The listing builds one solid part. Answer for the finished solid, in the listing's coordinates (mm). Give positions to 0.01 mm unless a question says otherwise; leave off trailing zeros. Loops run counter-clockwise (first coordinate to the right, second up) from the corner with the lowest first, then second, coordinate; pieces in that order, holes last. Notation, with made-up numbers: M 45,-31 L 60,-31 A21 ccw 60,-18 Z; hole C 56.5,1.25 d9. An arc over 180 degrees is marked long. One line per item, written item: value. Start each with the question number.
Q1. A cutting plane is placed at A-A, the plane x = -6. Determine the outline of the cut face in (y, z), and give its area (3 significant figures).
Q2. A cutting plane is placed at B-B, the plane y = -230. Determine the outline of the cut face in (x, z).
Q3. A cutting plane is placed at C-C, the plane z = 9. Determine the outline of the cut face in (x, y), and give its area (3 significant figures).
Q4. Consider L1, parallel to X at y = 451, z = 4; L2, parallel to Z at x = -18.5, y = 475.5. Determine where each line is inside the solid, lowest interval first.
from build123d import *

# Parameters (mm, degrees)
F0_W     = 50.8
F0_H     = 50.8
F0_W_2   = 41.275
F0_H_2   = 41.275
F1_DEPTH = 584.2
F3_DEPTH = 50.8
F4_R     = 5.08


with BuildPart() as f1:
    # F0 (on Front) → F1 (new body, symmetric)
    with BuildSketch(Plane.XZ):
        Rectangle(F0_W, F0_H)
        Rectangle(F0_W_2, F0_H_2, mode=Mode.SUBTRACT)
    extrude(amount=F1_DEPTH, both=True)

    # F2 (on face) → F3 (cut)
    with BuildSketch(Plane.YZ.offset(25.4)):
        Polygon((-584.2, 25.4), (-584.2, -25.4), (-535.14301, 25.4), align=None)
    extrude(amount=-F3_DEPTH, mode=Mode.SUBTRACT)

    # F4
    f4_edges = [f1.edges().sort_by_distance(p)[0] for p in [
        (-25.4, 24.528495, 25.4),
        (25.4, 24.528495, 25.4),
        (20.6375, 2.299546, -20.6375),
        (-20.6375, 2.299546, -20.6375),
        (-25.4, 0, -25.4),
        (25.4, 0, -25.4),
    ]]
    fillet(f4_edges, radius=F4_R)


solid = f1.part
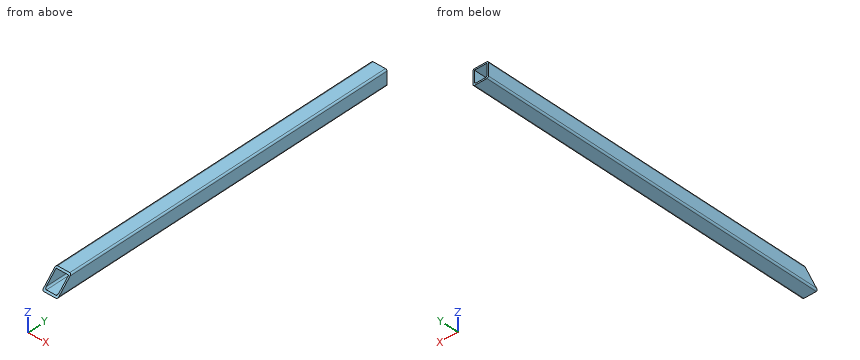
Answer block:
1. outline: M -584.2,-25.4 L 584.2,-25.4 L 584.2,-20.64 L -579.6,-20.64 Z; M -539.74,20.64 L 584.2,20.64 L 584.2,25.4 L -535.14,25.4 Z
1. area: 10,900 mm^2
2. outline: M -25.4,-20.32 A5.08 ccw -20.32,-25.4 L 20.32,-25.4 A5.08 ccw 25.4,-20.32 L 25.4,20.32 A5.08 ccw 20.32,25.4 L -20.32,25.4 A5.08 ccw -25.4,20.32 Z; hole M -20.64,-15.56 A5.08 ccw -15.56,-20.64 L 15.56,-20.64 A5.08 ccw 20.64,-15.56 L 20.64,20.64 L -20.64,20.64 Z
3. outline: M -25.4,-550.98 L -20.64,-550.98 L -20.64,584.2 L -25.4,584.2 Z; M 20.64,-550.98 L 25.4,-550.98 L 25.4,584.2 L 20.64,584.2 Z
3. area: 10,800 mm^2
4. L1: -25.4 to -20.64, 20.64 to 25.4
4. L2: -25.4 to -19.7, 20.64 to 25.4
